from build123d import *

# Parameters (mm, degrees)
BOSS_EXTRUDE1_DEPTH = 50.8
SKETCH2_W           = 30.48
SKETCH2_H           = 50.8
SKETCH2_R           = 3.175
SKETCH2_R_2         = 6.604
BOSS_EXTRUDE2_DEPTH = 5.08
SKETCH3_W           = 76.2
SKETCH3_H           = 25.4
CUT_EXTRUDE1_DEPTH  = 77.2
CUT_EXTRUDE2_DEPTH  = 51.8
BOSS_EXTRUDE3_DEPTH = 5.08
SKETCH6_R           = 16.51
CUT_EXTRUDE3_DEPTH  = 77.2


with BuildPart() as part:
    # Sketch1 → Boss-Extrude1 (new body, symmetric)
    with BuildSketch(Plane(origin=(0, 0, 0), x_dir=(0, 0, -1), z_dir=(1, 0, 0))):
        Polygon((-25.4, 0), (-20.32, 0), (-20.32, 71.12), (0, 71.12), (0, 76.2), (-25.4, 76.2), (-25.4, 71.12), align=None)
        Polygon((0, 76.2), (0, 71.12), (20.32, 71.12), (20.32, 0), (25.4, 0), (25.4, 71.12), (25.4, 76.2), align=None)
    extrude(amount=BOSS_EXTRUDE1_DEPTH, both=True)

    # Sketch2 → Boss-Extrude2 (add)
    with BuildSketch(Plane(origin=(0, 76.2, 0), x_dir=(1, 0, 0), z_dir=(0, 1, 0))):
        with Locations((-66.04, 0)):
            Rectangle(SKETCH2_W, SKETCH2_H)
        with Locations((-73.66, -12.7)):
            Circle(SKETCH2_R, mode=Mode.SUBTRACT)
        with Locations((-73.66, 12.7)):
            Circle(SKETCH2_R, mode=Mode.SUBTRACT)
        with BuildLine():
            Line((64.008, 12.7), (50.8, 12.7))
            Line((50.8, 12.7), (50.8, -12.7))
            Line((50.8, -12.7), (64.008, -12.7))
            ThreePointArc((64.008, -12.7), (76.708, 0), (64.008, 12.7))
        make_face()
        with Locations((64.008, 0)):
            Circle(SKETCH2_R_2, mode=Mode.SUBTRACT)
    extrude(amount=-BOSS_EXTRUDE2_DEPTH)

    # Sketch3 → Cut-Extrude1 (cut, through all)
    with BuildSketch(Plane(origin=(0, 76.2, 0), x_dir=(1, 0, 0), z_dir=(0, 1, 0))):
        with Locations((-12.7, 0)):
            Rectangle(SKETCH3_W, SKETCH3_H)
    extrude(amount=-CUT_EXTRUDE1_DEPTH, mode=Mode.SUBTRACT)

    # Sketch5 → Cut-Extrude2 (cut, through all)
    with BuildSketch(Plane.XY.offset(25.4)):
        Polygon((-25.4, 0), (-50.8, 71.12), (-50.8, 0), align=None)
        Polygon((50.8, 71.12), (25.4, 0), (50.8, 0), align=None)
    extrude(amount=-CUT_EXTRUDE2_DEPTH, mode=Mode.SUBTRACT)

    # Sketch4 → Boss-Extrude3 (add)
    with BuildSketch(Plane(origin=(0, 0, 0), x_dir=(-1, 0, 0), z_dir=(0, -1, 0))):
        with BuildLine():
            Line((-28.398063314, -25.4), (-43.994090512, -25.4))
            ThreePointArc((-43.994090512, -25.4), (0, -50.8), (43.994090512, -25.4))
            Line((43.994090512, -25.4), (28.398063314, -25.4))
            ThreePointArc((28.398063314, -25.4), (17.387076227, -33.901321217), (4.058215973, -37.883253333))
            ThreePointArc((4.058215973, -37.883253333), (4.062553736, -37.991588086), (4.064, -38.1))
            ThreePointArc((4.064, -38.1), (-0.108411914, -42.162553736), (-4.058215973, -37.883253333))
            ThreePointArc((-4.058215973, -37.883253333), (-17.387076227, -33.901321217), (-28.398063314, -25.4))
        make_face()
        with BuildLine():
            ThreePointArc((46.558969061, -20.32), (49.728440697, -10.378929899), (50.8, 0))
            ThreePointArc((50.8, 0), (-10.378929899, 49.728440697), (-46.558969061, -20.32))
            Line((-46.558969061, -20.32), (-32.228986953, -20.32))
            ThreePointArc((-32.228986953, -20.32), (-35.986705384, -12.512674997), (-37.883253333, -4.058215973))
            ThreePointArc((-37.883253333, -4.058215973), (-42.164, 0), (-37.883253333, 4.058215973))
            ThreePointArc((-37.883253333, 4.058215973), (-26.940768363, 26.940768363), (-4.058215973, 37.883253333))
            ThreePointArc((-4.058215973, 37.883253333), (-0.108411914, 42.162553736), (4.064, 38.1))
            ThreePointArc((4.064, 38.1), (4.062553736, 37.991588086), (4.058215973, 37.883253333))
            ThreePointArc((4.058215973, 37.883253333), (26.940768363, 26.940768363), (37.883253333, 4.058215973))
            ThreePointArc((37.883253333, 4.058215973), (40.896000496, 2.949318095), (42.164, 0))
            ThreePointArc((42.164, 0), (40.896000496, -2.949318095), (37.883253333, -4.058215973))
            ThreePointArc((37.883253333, -4.058215973), (35.986705384, -12.512674997), (32.228986953, -20.32))
            Line((32.228986953, -20.32), (46.558969061, -20.32))
        make_face()
        with BuildLine():
            ThreePointArc((-37.883253333, -4.058215973), (-35.986705384, -12.512674997), (-32.228986953, -20.32))
            Line((-32.228986953, -20.32), (32.228986953, -20.32))
            ThreePointArc((32.228986953, -20.32), (35.986705384, -12.512674997), (37.883253333, -4.058215973))
            ThreePointArc((37.883253333, -4.058215973), (34.036, 0), (37.883253333, 4.058215973))
            ThreePointArc((37.883253333, 4.058215973), (26.940768363, 26.940768363), (4.058215973, 37.883253333))
            ThreePointArc((4.058215973, 37.883253333), (0, 34.036), (-4.058215973, 37.883253333))
            ThreePointArc((-4.058215973, 37.883253333), (-26.940768363, 26.940768363), (-37.883253333, 4.058215973))
            ThreePointArc((-37.883253333, 4.058215973), (-35.150681905, 2.796000496), (-34.036, 0))
            ThreePointArc((-34.036, 0), (-35.150681905, -2.796000496), (-37.883253333, -4.058215973))
        make_face()
        with BuildLine():
            Line((-32.228986953, -20.32), (-46.558969061, -20.32))
            ThreePointArc((-46.558969061, -20.32), (-45.347720444, -22.895943975), (-43.994090512, -25.4))
            Line((-43.994090512, -25.4), (-28.398063314, -25.4))
            ThreePointArc((-28.398063314, -25.4), (-30.41975355, -22.940108848), (-32.228986953, -20.32))
        make_face()
        with BuildLine():
            ThreePointArc((43.994090512, -25.4), (45.347720444, -22.895943975), (46.558969061, -20.32))
            Line((46.558969061, -20.32), (32.228986953, -20.32))
            ThreePointArc((32.228986953, -20.32), (30.41975355, -22.940108848), (28.398063314, -25.4))
            Line((28.398063314, -25.4), (43.994090512, -25.4))
        make_face()
        with BuildLine():
            Line((28.398063314, -25.4), (-28.398063314, -25.4))
            ThreePointArc((-28.398063314, -25.4), (-17.387076227, -33.901321217), (-4.058215973, -37.883253333))
            ThreePointArc((-4.058215973, -37.883253333), (0, -34.036), (4.058215973, -37.883253333))
            ThreePointArc((4.058215973, -37.883253333), (17.387076227, -33.901321217), (28.398063314, -25.4))
        make_face()
        with BuildLine():
            Line((32.228986953, -20.32), (-32.228986953, -20.32))
            ThreePointArc((-32.228986953, -20.32), (-30.41975355, -22.940108848), (-28.398063314, -25.4))
            Line((-28.398063314, -25.4), (28.398063314, -25.4))
            ThreePointArc((28.398063314, -25.4), (30.41975355, -22.940108848), (32.228986953, -20.32))
        make_face()
    extrude(amount=BOSS_EXTRUDE3_DEPTH)

    # Sketch6 → Cut-Extrude3 (cut, through all)
    with BuildSketch(Plane.XY.offset(25.4)):
        with Locations((0, 38.1)):
            Circle(SKETCH6_R)
    extrude(amount=-CUT_EXTRUDE3_DEPTH, mode=Mode.SUBTRACT)


solid = part.part
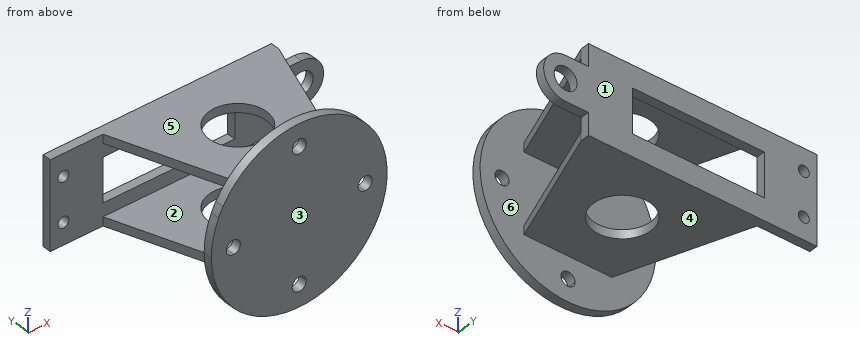
CAD build for the part. Positions are in the model's coordinates, mm. Face numbers are marked on the shaded views. A direction names the side the tool comes from. Give positions to 0.01 mm unless a question says otherwise; leave off trailing zeros. Write each loop counter-clockwise with the first axis right and the second up, starting at its lowest first coordinate (ties: lowest second). Pieces come first, ordered by that corner, then holes. Notation, with made-up numbers: M 45,-6 L 63,-6 A29 ccw 63,25 Z; hole C -4,70 d2. An arc over 180 degrees is marked long. Put each result on its own line as item: value. Start each with the question number.
(1) Band-saw the part on A-A, the plane y = 7. Write the cut outline in (x, z).
(2) Flat gauge pins, fed straight in: pin 1 Ø5.5 at (x, y) = (55.5, 73) entering from -Z; pin 2 Ø10 at (y, z) = (55, -14.5) entering from -X; pin 3 Ø1.5 at (x, y) = (55.5, 72.5) entering from +Z; pin 4 Ø7.5 at (x, z) = (-73.66, 12.7) entering from -Y. Where does each tip first touch, or does it go through?
(3) Mould opens along Z. For the marked faces 3, 4, 5 and 6 say: +Z half, -Z half, draft (parallel to the pull), parting line (faces both ways), or undercut.
(4) Which spindle directions (+Z, -Z, +X, -X, +Y, -Y) get a long thin tool onto all of the face, cutting with end or side? Do the marked faces 1 and 2. Say none if no direction does.
(5) Probe L1, parallel to X at y = 73.7, z = 0; L2, parallel to Y at x = 0, z = -22; L3, parallel to Z at x = -25, y = 1. List the from-to ranges inside material, lowest first.
(6) Band-saw the part on C-C, the plane z = -2. Write the cut outline in (x, y), and give its area (3 significant figures).
(7) Band-saw the part on D-D, the plane z = -23. Write the cut outline in (x, y).
(8) Band-saw the part on B-B, the plane x = -73.66. Write the cut outline in (y, z) (3 decimals).
Response values:
1. outline: M -27.9,-25.4 L 27.9,-25.4 L 27.9,-20.32 L -27.9,-20.32 Z; M -27.9,20.32 L 27.9,20.32 L 27.9,25.4 L -27.9,25.4 Z
2. pin 1: stops at z = -12.7
2. pin 2: passes through
2. pin 3: stops at z = 12.7
2. pin 4: stops at y = 71.12
3. face 3: draft
3. face 4: -Z half
3. face 5: +Z half
3. face 6: undercut
4. face 1: +Z, -Z, +X, -X, +Y
4. face 2: +X, -X
5. L1: x = -81.28 to -50.8, 25.4 to 57.4, 70.61 to 76.71
5. L2: y = -5.08 to 21.59, 54.61 to 76.2
5. L3: z = -25.4 to -20.32, 20.32 to 25.4
6. outline: M -81.28,71.12 L -50.8,71.12 L -50.8,76.2 L -81.28,76.2 Z; M -50.76,-5.08 L -41.64,-5.08 L -41.64,0 L -50.76,0 Z; M -34.56,-5.08 L 34.56,-5.08 L 34.56,0 L -34.56,0 Z; M 25.4,71.12 L 57.71,71.12 L 57.71,76.2 L 25.4,76.2 Z; M 41.64,-5.08 L 50.76,-5.08 L 50.76,0 L 41.64,0 Z; M 70.3,71.12 L 76.55,71.12 L 76.55,76.2 L 70.3,76.2 Z
6. area: 795 mm2
7. outline: M -81.28,71.12 L -50.8,71.12 L -25.4,0 L -45.3,0 L -45.3,-5.08 L 45.3,-5.08 L 45.3,0 L 25.4,0 L 50.8,71.12 L 50.8,76.2 L -81.28,76.2 Z; hole C 0,38.1 d33.02
8. outline: M 71.12,-25.4 L 76.2,-25.4 L 76.2,-15.875 L 71.12,-15.875 Z; M 71.12,-9.525 L 76.2,-9.525 L 76.2,9.525 L 71.12,9.525 Z; M 71.12,15.875 L 76.2,15.875 L 76.2,25.4 L 71.12,25.4 Z
